Verification items for the finished model (mm, model axes). A direction names the side the tool comes from. Round coordinates to 2 decimals unless told otherwise and drop trailing zeros. Write each loop counter-clockwise with the first axis right and the second up, starting at its lowest first coordinate (ties: lowest second). Pieces come first, ordered by that corner, then holes. Notation, with made-up numbers: M 59.5,59 L 83.5,59 A24 cw 83.5,88 Z; hole C 77.5,2.25 d8. An arc over 180 degrees is marked long. Answer in a Markdown table with one row per item. Add a question column.
1. Set-up check for faces 5 (the flat face through (-6, 0, -2)), 6 (the flat face through (-6, 38.5, 92)): record each of +Z, -Z, +X, -X, +Y, -Y from which the full face is reachable in a straight line by a thin tool's end or side.
2. Sectioned sample at C-C on z = 43. Record the cut outline in (x, y), plus the area to 3 significant figures.
3. Sectioned sample at A-A on x = 296. Record the cut outline in (y, z).
4. Material ranges on probe 1 along Z at (x, y) = (310, 17.5); probe 2 along Y at (x, z) = (-142, 98.5); probe 3 along Y at (x, z) = (-375, -63), recorded low to high.
5. Sectioned sample at B-B on y = 18.5. Count the separate pieces of the cut face and the enclosed holes in it, plus the area to 3 significant figures.
6. Go/stop test with flat-tipped pins: pin 1 Ø1.2 at (x, y) = (-39, 38) entering from -Z; pin 2 Ø7 at (x, y) = (-380, 18.5) entering from +Z; pin 3 Ø7 at (x, z) = (228, 91.75) entering from +Y. Record where each tip stops, or that it passes through.
7. Draft check along X on faces 1 (the cylindrical face through (360.476, -0.74, -4.336)), 2 (the flat face through (-6, -1.5, -2)), 3 (the flat face through (460, -1, 1)), 4 (the flat face through (-460, -1, 1)). Enter one of: pulls with the +X half, pulls with the -X half, needs draft (parallel to the pull), parting line crosses it, or undercut.
```python
from build123d import *

# Parameters (mm, degrees)
SKETCH1_W                      = 920
SKETCH1_H                      = 225
BASE_FLANGE1_DEPTH             = 1.5
EDGE_FLANGE1_STRIP_W           = 10
EDGE_FLANGE1_STRIP_H           = 1.5
EDGE_FLANGE1_STRIP_CUT_DEPTH   = 920
EDGE_FLANGE1_STRIP_2_W         = 10
EDGE_FLANGE1_STRIP_2_H         = 1.5
EDGE_FLANGE1_STRIP_CUT_2_DEPTH = 920
EDGE_FLANGE1_DEPTH             = 920
EDGE_FLANGE1_BEND_DEPTH        = 920
EDGE_FLANGE2_STRIP_W           = 10
EDGE_FLANGE2_STRIP_H           = 1.5
EDGE_FLANGE2_STRIP_CUT_DEPTH   = 920
EDGE_FLANGE2_STRIP_2_W         = 10
EDGE_FLANGE2_STRIP_2_H         = 1.5
EDGE_FLANGE2_STRIP_CUT_2_DEPTH = 920
EDGE_FLANGE2_DEPTH             = 920
EDGE_FLANGE2_BEND_DEPTH        = 920
SKETCH18_R                     = 6
CUT_EXTRUDE1_DEPTH             = 280
SKETCH19_R                     = 6
CUT_EXTRUDE2_DEPTH             = 5
SKETCH20_R                     = 20
CUT_EXTRUDE3_DEPTH             = 65


# Sheet-metal steps are written as plain solids
with BuildPart() as part:
    # Sketch1 → Base-Flange1 (new body)
    with BuildSketch(Plane(origin=(0, 0, 0), x_dir=(1, 0, 0), z_dir=(0, 1, 0))):
        Rectangle(SKETCH1_W, SKETCH1_H)
    extrude(amount=-BASE_FLANGE1_DEPTH)

    # Edge-Flange1 strip (across the edge) → Edge-Flange1 strip cut (cut)
    with BuildSketch(Plane(origin=(-460, 0, 112.5), x_dir=(0, 0, -1), z_dir=(1, 0, 0))):
        with Locations((-1.5, -0.75)):
            Rectangle(EDGE_FLANGE1_STRIP_W, EDGE_FLANGE1_STRIP_H)
    extrude(amount=EDGE_FLANGE1_STRIP_CUT_DEPTH, mode=Mode.SUBTRACT)

    # Edge-Flange1 strip 2 (across the edge) → Edge-Flange1 strip cut 2 (cut)
    with BuildSketch(Plane(origin=(460, 0, -112.5), x_dir=(0, 0, 1), z_dir=(-1, 0, 0))):
        with Locations((-1.5, -0.75)):
            Rectangle(EDGE_FLANGE1_STRIP_2_W, EDGE_FLANGE1_STRIP_2_H)
    extrude(amount=EDGE_FLANGE1_STRIP_CUT_2_DEPTH, mode=Mode.SUBTRACT)

    # Edge-Flange1 section (across the edge) → Edge-Flange1 (add)
    with BuildSketch(Plane(origin=(-460, 0, 112.5), x_dir=(0, 0, -1), z_dir=(1, 0, 0))):
        with BuildLine():
            Line((0, 2), (0, 38.5))
            Line((0, 38.5), (1.5, 38.5))
            Line((1.5, 38.5), (1.5, 2))
            ThreePointArc((1.5, 2), (2.085786438, 0.585786438), (3.5, 0))
            Line((3.5, 0), (3.5, -1.5))
            ThreePointArc((3.5, -1.5), (1.025126266, -0.474873734), (0, 2))
        make_face()
    extrude(amount=EDGE_FLANGE1_DEPTH)

    # Edge-Flange1 section 2 (across the edge) → Edge-Flange1 bend (add)
    with BuildSketch(Plane(origin=(460, 0, -112.5), x_dir=(0, 0, 1), z_dir=(-1, 0, 0))):
        with BuildLine():
            Line((0, 2), (0, 38.5))
            Line((0, 38.5), (1.5, 38.5))
            Line((1.5, 38.5), (1.5, 2))
            ThreePointArc((1.5, 2), (2.085786438, 0.585786438), (3.5, 0))
            Line((3.5, 0), (3.5, -1.5))
            ThreePointArc((3.5, -1.5), (1.025126266, -0.474873734), (0, 2))
        make_face()
    extrude(amount=EDGE_FLANGE1_BEND_DEPTH)

    # Edge-Flange2 strip (across the edge) → Edge-Flange2 strip cut (cut)
    with BuildSketch(Plane(origin=(-460, 38.5, 111), x_dir=(0, -1, 0), z_dir=(1, 0, 0))):
        with Locations((-1.5, -0.75)):
            Rectangle(EDGE_FLANGE2_STRIP_W, EDGE_FLANGE2_STRIP_H)
    extrude(amount=EDGE_FLANGE2_STRIP_CUT_DEPTH, mode=Mode.SUBTRACT)

    # Edge-Flange2 strip 2 (across the edge) → Edge-Flange2 strip cut 2 (cut)
    with BuildSketch(Plane(origin=(460, 38.5, -111), x_dir=(0, -1, 0), z_dir=(-1, 0, 0))):
        with Locations((-1.5, -0.75)):
            Rectangle(EDGE_FLANGE2_STRIP_2_W, EDGE_FLANGE2_STRIP_2_H)
    extrude(amount=EDGE_FLANGE2_STRIP_CUT_2_DEPTH, mode=Mode.SUBTRACT)

    # Edge-Flange2 section (across the edge) → Edge-Flange2 (add)
    with BuildSketch(Plane(origin=(-460, 38.5, 111), x_dir=(0, -1, 0), z_dir=(1, 0, 0))):
        with BuildLine():
            Line((0, 2), (0, 36.5))
            Line((0, 36.5), (1.5, 36.5))
            Line((1.5, 36.5), (1.5, 2))
            ThreePointArc((1.5, 2), (2.085786438, 0.585786438), (3.5, 0))
            Line((3.5, 0), (3.5, -1.5))
            ThreePointArc((3.5, -1.5), (1.025126266, -0.474873734), (0, 2))
        make_face()
    extrude(amount=EDGE_FLANGE2_DEPTH)

    # Edge-Flange2 section 2 (across the edge) → Edge-Flange2 bend (add)
    with BuildSketch(Plane(origin=(460, 38.5, -111), x_dir=(0, -1, 0), z_dir=(-1, 0, 0))):
        with BuildLine():
            Line((0, 2), (0, 36.5))
            Line((0, 36.5), (1.5, 36.5))
            Line((1.5, 36.5), (1.5, 2))
            ThreePointArc((1.5, 2), (2.085786438, 0.585786438), (3.5, 0))
            Line((3.5, 0), (3.5, -1.5))
            ThreePointArc((3.5, -1.5), (1.025126266, -0.474873734), (0, 2))
        make_face()
    extrude(amount=EDGE_FLANGE2_BEND_DEPTH)

    # Sketch18 → Cut-Extrude1 (cut)
    with BuildSketch(Plane.XY.offset(112.5)):
        with Locations((380, 18.5)):
            Circle(SKETCH18_R)
        with Locations((228, 18.5)):
            Circle(SKETCH18_R)
        with Locations((76, 18.5)):
            Circle(SKETCH18_R)
        with Locations((-76, 18.5)):
            Circle(SKETCH18_R)
        with Locations((-228, 18.5)):
            Circle(SKETCH18_R)
        with Locations((-380, 18.5)):
            Circle(SKETCH18_R)
    extrude(amount=-CUT_EXTRUDE1_DEPTH, mode=Mode.SUBTRACT)

    # Sketch19 → Cut-Extrude2 (cut)
    with BuildSketch(Plane(origin=(0, 38.5, 0), x_dir=(1, 0, 0), z_dir=(0, 1, 0))):
        with Locations(Location((-380, -91.75, 0), (0, 0, 270))):
            Circle(SKETCH19_R)
        with Locations(Location((-228, -91.75, 0), (0, 0, 270))):
            Circle(SKETCH19_R)
        with Locations(Location((-76, -91.75, 0), (0, 0, 270))):
            Circle(SKETCH19_R)
        with Locations(Location((76, -91.75, 0), (0, 0, 270))):
            Circle(SKETCH19_R)
        with Locations(Location((228, -91.75, 0), (0, 0, 270))):
            Circle(SKETCH19_R)
        with Locations(Location((380, -91.75, 0), (0, 0, 270))):
            Circle(SKETCH19_R)
        with Locations(Location((380, 91.75, 0), (0, 0, 90))):
            Circle(SKETCH19_R)
        with Locations(Location((228, 91.75, 0), (0, 0, 90))):
            Circle(SKETCH19_R)
        with Locations(Location((76, 91.75, 0), (0, 0, 90))):
            Circle(SKETCH19_R)
        with Locations(Location((-76, 91.75, 0), (0, 0, 90))):
            Circle(SKETCH19_R)
        with Locations(Location((-228, 91.75, 0), (0, 0, 90))):
            Circle(SKETCH19_R)
        with Locations(Location((-380, 91.75, 0), (0, 0, 90))):
            Circle(SKETCH19_R)
    extrude(amount=-CUT_EXTRUDE2_DEPTH, mode=Mode.SUBTRACT)

    # Sketch20 → Cut-Extrude3 (cut)
    with BuildSketch(Plane(origin=(0, 0, 0), x_dir=(1, 0, 0), z_dir=(0, 1, 0))):
        with Locations(Location((-380, 0, 0), (0, 0, 270))):
            Circle(SKETCH20_R)
        with Locations(Location((-228, 0, 0), (0, 0, 270))):
            Circle(SKETCH20_R)
        with Locations(Location((-76, 0, 0), (0, 0, 270))):
            Circle(SKETCH20_R)
        with Locations(Location((76, 0, 0), (0, 0, 270))):
            Circle(SKETCH20_R)
        with Locations(Location((228, 0, 0), (0, 0, 270))):
            Circle(SKETCH20_R)
        with Locations(Location((380, 0, 0), (0, 0, 270))):
            Circle(SKETCH20_R)
    extrude(amount=-CUT_EXTRUDE3_DEPTH, mode=Mode.SUBTRACT)


solid = part.part
```
Geometry check:
| question | item | result |
|---|---|---|
| 1 | face 5 | +X, -X |
| 1 | face 6 | +Z, -Z, +X, -X, +Y |
| 2 | outline | M -460,-1.5 L 460,-1.5 L 460,0 L -460,0 Z |
| 2 | area | 1,380 mm2 |
| 3 | outline | M -1.5,-109 A3.5 ccw 2,-112.5 L 35,-112.5 A3.5 ccw 38.5,-109 L 38.5,-74.5 L 37,-74.5 L 37,-109 A2 cw 35,-111 L 2,-111 A2 cw 0,-109 L 0,109 A2 cw 2,111 L 35,111 A2 cw 37,109 L 37,74.5 L 38.5,74.5 L 38.5,109 A3.5 ccw 35,112.5 L 2,112.5 A3.5 ccw -1.5,109 Z |
| 4 | probe 1 | z = -112.5 to -111, 111 to 112.5 |
| 4 | probe 2 | y = -1.5 to 0, 37 to 38.5 |
| 4 | probe 3 | y = -1.5 to 0 |
| 5 | separate pieces | 14 |
| 5 | enclosed holes | 0 |
| 5 | area | 2,540 mm2 |
| 6 | pin 1 | stops at z = -111.55 |
| 6 | pin 2 | passes through |
| 6 | pin 3 | stops at y = 0 |
| 7 | face 1 | undercut |
| 7 | face 2 | needs draft |
| 7 | face 3 | pulls with the +X half |
| 7 | face 4 | pulls with the -X half |
